```python
from build123d import *

# Parameters (mm, degrees)
F0_W     = 0.75
F0_H     = 0.5
F0_R     = 0.5
F0_R_2   = 0.625
F1_DEPTH = 1.9


# Not quite as in the source:
# - ends of sketch curves that miss each other by under 0.0002 mm in the source are joined


with BuildPart() as f1:
    # F0 (on Front) → F1 (new body)
    with BuildSketch(Plane.XZ):
        with BuildLine():
            Line((0.0021614751, 1.1225641938), (1.122697085, 0.0020285839))
            Line((1.122697085, 0.0020285839), (3.625, 0.0020285839))
            ThreePointArc((3.625, 0.0020285839), (3.8901650429, -0.1078063731), (4, -0.3729714161))
            Line((4, -0.3729714161), (4, -1.4979714161))
            Line((4, -1.4979714161), (6.0021614751, -1.4979714161))
            Line((6.0021614751, -1.4979714161), (6.0021614751, 0.5020285839))
            Line((6.0021614751, 0.5020285839), (7.2521614751, 1.7551845998))
            Line((7.2521614751, 1.7551845998), (7.2521614751, 3))
            Line((7.2521614751, 3), (7.2521614751, 3.0051845998))
            ThreePointArc((7.2521614751, 3.0051845998), (5.9995691919, 4.249997312), (4.7521614751, 3))
            Line((4.7521614751, 3), (4.7521614751, 2.375))
            ThreePointArc((4.7521614751, 2.375), (4.642326518, 2.1098349571), (4.3771614751, 2))
            Line((4.3771614751, 2), (2.3771614751, 2))
            ThreePointArc((2.3771614751, 2), (2.1119964322, 2.1098349571), (2.0021614751, 2.375))
            Line((2.0021614751, 2.375), (2.0021614751, 3))
            ThreePointArc((2.0021614751, 3), (1.0021614751, 4), (0.0021614751, 3))
            Line((0.0021614751, 3), (0.0021614751, 1.1225641938))
        make_face()
        with BuildLine():
            ThreePointArc((5.3746090938, -0.9511214132), (4.9914239554, -1.3089053091), (4.6250000012, -0.9339737791))
            Line((4.6250000012, -0.9339737791), (4.6250586901, -0.1906377023))
            ThreePointArc((4.6250586901, -0.1906377023), (5.0052444867, 0.1909599387), (5.3746090938, -0.2011214132))
            Line((5.3746090938, -0.2011214132), (5.3746090938, -0.9168853601))
            ThreePointArc((5.3746090938, -0.9168853601), (5.375, -0.9340033866), (5.3746090938, -0.9511214132))
        make_face(mode=Mode.SUBTRACT)
        with Locations((1.6271614751, 1.5020285839)):
            Rectangle(F0_W, F0_H, mode=Mode.SUBTRACT)
        with Locations((1.0021614751, 3)):
            Circle(F0_R, mode=Mode.SUBTRACT)
        with Locations((6.0021614751, 3)):
            Circle(F0_R_2, mode=Mode.SUBTRACT)
    extrude(amount=F1_DEPTH)


solid = f1.part
```
The model under review builds one solid part; all positions refer to its coordinate system, in mm. A direction names the side the tool comes from. Round coordinates to 2 decimals unless told otherwise and drop trailing zeros. Loops run counter-clockwise (first coordinate to the right, second up) from the corner with the lowest first, then second, coordinate; pieces in that order, holes last. Notation, with made-up numbers: M -34,56 L -1,56 A6 ccw -1,65 Z; hole C 71,-9.5 d5. An arc over 180 degrees is marked long. Write item = value, one per line.
Item 1: For line 1 (X direction, y = -1.7, z = -0.95); line 2 (Z direction, x = 3.5, y = -1.1); line 3 (X direction, y = -0.5, z = 3.2), list the stretches that pass through material, from the lowest coordinate up. Write a range as [from, to].
Return value:
line_1 = [4, 4.63], [5.37, 6]
line_2 = [0, 2]
line_3 = [0.02, 0.54], [1.46, 1.98], [4.77, 5.41], [6.59, 7.24]
Item 2: Take a section at B-B on x = 0.75. Write out the cut boundary in (y, z), then the cut area to 3 significant figures.
Return value:
outline = M -1.9,0.37 L 0,0.37 L 0,2.57 L -1.9,2.57 Z; M -1.9,3.43 L 0,3.43 L 0,3.97 L -1.9,3.97 Z
area = 5.19 mm2
Item 3: Machinability: for faces 1 (the flat face through (6.002, -1, -1)), 2 (the flat face through (4, -1.9, 1)), 3 (the flat face through (2, -1, 0.002)), which of the approach directions +Z, -Z, +X, -X, +Y, -Y give a long, thin tool a straight path to every point of the face, cutting with its end or side? Answer none if there is none.
Return value:
face_1 = -Z, +X, +Y, -Y
face_2 = +Z, -Z, +X, -X, -Y
face_3 = -Z, -X, +Y, -Y
Item 4: Take a section at C-C on x = 3.5. Write out the cut boundary in (y, z).
Return value:
outline = M -1.9,0 L 0,0 L 0,2 L -1.9,2 Z
Item 5: Take a section at A-A on y = -1.1. Write out the cut boundary in (x, z) (3 decimals), then the cut area to 3 significant figures.
Return value:
outline = M 0.002,1.123 L 1.123,0.002 L 3.625,0.002 A0.375 cw 4,-0.373 L 4,-1.498 L 6.002,-1.498 L 6.002,0.502 L 7.252,1.755 L 7.252,3.005 A1.25 ccw 4.752,3 L 4.752,2.375 A0.375 cw 4.377,2 L 2.377,2 A0.375 cw 2.002,2.375 L 2.002,3 A1 ccw 0.002,3 Z; hole C 1.002,3 d1; hole M 1.252,1.252 L 2.002,1.252 L 2.002,1.752 L 1.252,1.752 Z; hole M 4.625,-0.934 A0.375 ccw long 5.375,-0.917 L 5.375,-0.201 A0.375 ccw long 4.625,-0.191 Z; hole C 6.002,3 d1.25
area = 20.7 mm2
Item 6: The part is to be moulded in two halves that separate along X. For faces 4 (the flat face through (0.555, -0.937, 0.57)), 5 (the flat face through (3, -1, 2)), 6 (the flat face through (5, -1, -1.498)), say which applies: released by +X, released by -X, zero draft, split by the parting line, or undercut.
Return value:
face_4 = released by -X
face_5 = undercut
face_6 = zero draft
Item 7: Take a section at D-D on x = 5. Write out the cut boundary in (y, z), then the cut area to 3 significant figures.
Return value:
outline = M -1.9,-1.5 L 0,-1.5 L 0,-1.31 L -1.9,-1.31 Z; M -1.9,0.19 L 0,0.19 L 0,3.75 L -1.9,3.75 Z
area = 7.12 mm2
Item 8: Insertion check: P1, Ø1, axis at x = 2, y = -1.5, coming from the -Z side; P2, Ø0.6, axis at y = -1.5, z = 1.5, coming from the +X side; P3, Ø0.9, axis at y = -1, z = -1, coming from the -X side; P4, Ø1, axis at x = 4.5, y = -0.5, coming from the +Z side. Each pin has a flat end and moves straight along its axis. Give the tip position at first contact, or say it passes through.
Return value:
P1 = 0
P2 = 7.25
P3 = 4
P4 = 3.75
